```python
from build123d import *

# Parameters (mm, degrees)
SKETCH_1_R      = 1.65
EXTRUDE_1_DEPTH = 3


with BuildPart() as part:
    # 草图1 → 凸台-拉伸1 (new body)
    with BuildSketch(Plane(origin=(0, 0, 0), x_dir=(1, 0, 0), z_dir=(0, 1, 0))):
        with BuildLine():
            Line((10, 0), (10, 30))
            Line((10, 30), (0, 30))
            ThreePointArc((0, 30), (-17.67766953, 37.32233047), (-25, 55))
            ThreePointArc((-25, 55), (-35, 65), (-45, 55))
            ThreePointArc((-45, 55), (-35.178118199, 26.937569599), (-10, 11.125178063))
            Line((-10, 11.125178063), (-10, 0))
            ThreePointArc((-10, 0), (0, -10), (10, 0))
        make_face()
        with Locations(Location((-35, 55, 0), (0, 0, 270))):
            Circle(SKETCH_1_R, mode=Mode.SUBTRACT)
        with Locations(Location((0, 20, 0), (0, 0, 270))):
            Circle(SKETCH_1_R, mode=Mode.SUBTRACT)
        with Locations(Location((0, 0, 0), (0, 0, 270))):
            Circle(SKETCH_1_R, mode=Mode.SUBTRACT)
    extrude(amount=EXTRUDE_1_DEPTH)


solid = part.part
```
The model under review builds one solid part; all positions refer to its coordinate system, in mm. A direction names the side the tool comes from. Round coordinates to 2 decimals unless told otherwise and drop trailing zeros. Loops run counter-clockwise (first coordinate to the right, second up) from the corner with the lowest first, then second, coordinate; pieces in that order, holes last. Notation, with made-up numbers: (21, 65) -> (33, 65) arc R26 ccw to (33, 93) -> close; hole circle Ø9 at (-29.75, 55.25). An arc over 180 degrees is marked (long way). Answer as a JSON object with one key per item and string values. Group by question number.
1) Mouldability with a two-part tool opening along Z and no side actions: class faces 1 (the face through (-18, 0, -28)), 2 (the face through (-33.885, 1.479, -56.216)), 3 (the face through (5, 1, -30)) as released by +Z, released by -Z, zero draft, split by the parting line, or undercut.
2) We need section A-A on y = 2. Write out the cut boundary in (x, z).
3) For line 1 (X direction, y = 0.6, z = -55); line 2 (X direction, y = 0.95, z = -20); line 3 (X direction, y = 0.5, z = -9.5), list the stretches that pass through material, from the lowest coordinate up. Write a range as [from, to].
4) We need section C-C on z = -20. Write out the cut boundary in (x, y).
5) We need section D-D on z = -33. Write out the cut boundary in (x, y).
6) For pin 1 Ø4 at (x, z) = (-35, -55) entering from -Y; pin 2 Ø1.5 at (y, z) = (1.5, -6.5) entering from -X; pin 3 Ø0.9 at (x, y) = (5, 2) entering from -Z; pin 4 Ø1 at (x, y) = (-34, 0.5) entering from -Z, all flat-tipped, find the tip position at first contact; note any pin that passes through.
7) For faces 4 (the face through (-10, 1, -6)), 5 (the face through (-35, 1, -65)), list the 3-axis set-ups (+Z, -Z, +X, -X, +Y, -Y) from which the entire face can be reached by the end or side of a thin tool; tool diameter is ignored.
8) We need section B-B on x = -35. Write out the cut boundary in (y, z), then the cut area to 3 significant figures.
Result set:
{
 "1": {"face 1": "zero draft", "face 2": "undercut", "face 3": "released by -Z"},
 "2": {"outline": "(-45, -55) arc R10 ccw to (-25, -55) arc R25 cw to (0, -30) -> (10, -30) -> (10, 0) arc R10 ccw to (-10, 0) -> (-10, -11.13) arc R45 ccw to start; hole circle Ø3.3 at (-35, -55); hole circle Ø3.3 at (0, -20); hole circle Ø3.3 at (0, 0)"},
 "3": {"line 1": "[-45, -36.65], [-33.35, -25]", "line 2": "[-28.28, -1.65], [1.65, 10]", "line 3": "[-10, 10]"},
 "4": {"outline": "(-28.28, 0) -> (-1.65, 0) -> (-1.65, 3) -> (-28.28, 3) -> close; (1.65, 0) -> (10, 0) -> (10, 3) -> (1.65, 3) -> close"},
 "5": {"outline": "(-39.26, 0) -> (-11.87, 0) -> (-11.87, 3) -> (-39.26, 3) -> close"},
 "6": {"pin 1": "y = 0", "pin 2": "x = -10", "pin 3": "z = -30", "pin 4": "z = -64.99"},
 "7": {"face 4": "+Z, -X, +Y, -Y", "face 5": "-Z, +Y, -Y"},
 "8": {"outline": "(0, -65) -> (3, -65) -> (3, -56.65) -> (0, -56.65) -> close; (0, -53.35) -> (3, -53.35) -> (3, -26.72) -> (0, -26.72) -> close", "area": "105 mm²"}
}
